Geometry: final body of the model. Coordinates: model frame, mm. Face numbers are marked on the shaded views. A direction names the side the tool comes from. Round coordinates to 2 decimals unless told otherwise and drop trailing zeros. Loops run counter-clockwise (first coordinate to the right, second up) from the corner with the lowest first, then second, coordinate; pieces in that order, holes last. Notation, with made-up numbers: (4.25, -18) - (53.25, -18) arc R16 cw to (53.25, 2) - close; hole circle Ø10 at (49.25, 81.5). An arc over 180 degrees is marked (long way). Write item = value, one per line. Start each with the question number.
Item 1: Line query: line 1 (Z direction, x = -1, y = -1.7); line 2 (Y direction, x = 0.5, z = 0.8); line 3 (Y direction, x = 2.5, z = -0.9). Output: solid intervals per line, ascending. Write a range as from..to.
Item 2: Section A-A (z = 0). Return loops of the section in (x, y).
Item 3: Section C-C (y = -0.75). Return loops of the section in (x, z) (3 decimals).
Item 4: First-contact query: pin 1 (0.6 mm diameter, centred on x = -3, y = 0, fed in from -Z); pin 2 (1.5 mm diameter, centred on x = -2.5, z = 0, fed in from +Y); pin 3 (1.2 mm diameter, centred on x = 0.5, z = 0, fed in from +Y); pin 4 (1 mm diameter, centred on x = -1.5, z = 2, fed in from -Y). Flat tips, straight axial feed; report the tip coordinate or a pass-through.
Item 5: Access query for the marked faces 4 and 5. Directions: +Z, -Z, +X, -X, +Y, -Y. A direction counts if a zero-diameter tool reaches every point of the face in a straight line with its end or side. Return the directions, or none.
Item 6: Draft query along Z for the marked faces 1, 2 and 3. Return one class per face: pulls with the +Z half, pulls with the -Z half, needs draft (parallel to the pull), parting line crosses it, or undercut.
Item 7: Section B-B (x = 0). Return loops of the section in (y, z).
Item 8: Section D-D (x = -2.75). Return loops of the section in (y, z).
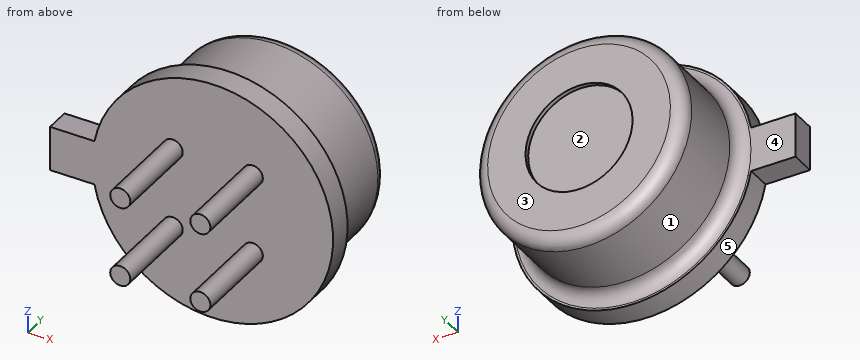
from build123d import *

# Parameters (mm, degrees)
SKETCH1_R           = 2.35
BOSS_EXTRUDE1_DEPTH = 2.6
SKETCH2_R           = 2.7
BOSS_EXTRUDE2_DEPTH = 0.55
FILLET1_R           = 0.3
FILLET2_R           = 0.3
SKETCH3_R           = 1.2
CUT_EXTRUDE1_DEPTH  = 0.1
SKETCH4_W           = 1.15
SKETCH4_H           = 1
BOSS_EXTRUDE3_DEPTH = 0.55
SKETCH5_R           = 0.225
BOSS_EXTRUDE4_DEPTH = 2


with BuildPart() as part:
    # Sketch1 → Boss-Extrude1 (new body)
    with BuildSketch(Plane(origin=(0, 0, 0), x_dir=(1, 0, 0), z_dir=(0, 1, 0))):
        with Locations(Location((0, 0, 0), (0, 0, 270))):
            Circle(SKETCH1_R)
    extrude(amount=BOSS_EXTRUDE1_DEPTH)

    # Sketch2 → Boss-Extrude2 (add)
    with BuildSketch(Plane.XZ):
        with Locations(Location((0, 0, 0), (0, 0, 270))):
            Circle(SKETCH2_R)
    extrude(amount=-BOSS_EXTRUDE2_DEPTH)

    # Fillet1
    fillet1_edges = [part.edges().sort_by_distance(p)[0] for p in [
        (0, 0.55, -2.35),
    ]]
    fillet(fillet1_edges, radius=FILLET1_R)

    # Fillet2
    fillet2_edges = [part.edges().sort_by_distance(p)[0] for p in [
        (0, 2.6, -2.35),
    ]]
    fillet(fillet2_edges, radius=FILLET2_R)

    # Sketch3 → Cut-Extrude1 (cut)
    with BuildSketch(Plane(origin=(0, 2.6, 0), x_dir=(1, 0, 0), z_dir=(0, 1, 0))):
        with Locations(Location((0, 0, 0), (0, 0, 270))):
            Circle(SKETCH3_R)
    extrude(amount=-CUT_EXTRUDE1_DEPTH, mode=Mode.SUBTRACT)

    # Sketch4 → Boss-Extrude3 (add)
    with BuildSketch(Plane.XZ):
        with Locations((-3.075, 0)):
            Rectangle(SKETCH4_W, SKETCH4_H)
    extrude(amount=-BOSS_EXTRUDE3_DEPTH)

    # Sketch5 → Boss-Extrude4 (add)
    with BuildSketch(Plane.XZ):
        with Locations(Location((-0.898025612, 0.898025612, 0), (0, 0, 90))):
            Circle(SKETCH5_R)
        with Locations(Location((0.898025612, 0.898025612, 0), (0, 0, 90))):
            Circle(SKETCH5_R)
        with Locations(Location((-0.898025612, -0.898025612, 0), (0, 0, 90))):
            Circle(SKETCH5_R)
        with Locations(Location((0.898025612, -0.898025612, 0), (0, 0, 90))):
            Circle(SKETCH5_R)
    extrude(amount=BOSS_EXTRUDE4_DEPTH)


solid = part.part
Taken from the geometry:
q1.line_1 = -1.1..-0.7, 0.7..1.1
q1.line_2 = 0..2.5
q1.line_3 = 0..0.55
q2.outline = (-3.65, 0) - (2.7, 0) - (2.7, 0.55) - (2.65, 0.55) arc R0.3 cw to (2.35, 0.85) - (2.35, 2.3) arc R0.3 ccw to (2.05, 2.6) - (1.2, 2.6) - (1.2, 2.5) - (-1.2, 2.5) - (-1.2, 2.6) - (-2.05, 2.6) arc R0.3 ccw to (-2.35, 2.3) - (-2.35, 0.85) arc R0.3 cw to (-2.65, 0.55) - (-3.65, 0.55) - close
q3.outline = circle Ø0.45 at (-0.898, -0.898); circle Ø0.45 at (-0.898, 0.898); circle Ø0.45 at (0.898, -0.898); circle Ø0.45 at (0.898, 0.898)
q4.pin_1 = -0.5
q4.pin_2 = 2.6
q4.pin_3 = 2.5
q4.pin_4 = 0
q5.face_4 = +Y
q5.face_5 = +Y, -Y
q6.face_1 = parting line crosses it
q6.face_2 = undercut
q6.face_3 = needs draft
q7.outline = (0, -2.7) - (0.55, -2.7) - (0.55, -2.65) arc R0.3 cw to (0.85, -2.35) - (2.3, -2.35) arc R0.3 ccw to (2.6, -2.05) - (2.6, -1.2) - (2.5, -1.2) - (2.5, 1.2) - (2.6, 1.2) - (2.6, 2.05) arc R0.3 ccw to (2.3, 2.35) - (0.85, 2.35) arc R0.3 cw to (0.55, 2.65) - (0.55, 2.7) - (0, 2.7) - close
q8.outline = (0, -0.5) - (0.55, -0.5) - (0.55, 0.5) - (0, 0.5) - close
